from build123d import *

# Parameters (mm, degrees)
F1_DEPTH  = 25.4
F2_R      = 3.556
F3_DEPTH  = 30.342798
F3_FACE_R = 3.556
F4_DEPTH  = 45.857202


with BuildPart() as f1:
    # F0 (on Top) → F1 (new body)
    with BuildSketch(Plane.XY):
        with BuildLine():
            Line((-2.147933, 7.757202), (-29.198933, 7.757202))
            Line((-29.198933, 7.757202), (-29.198933, -30.342798))
            Line((-29.198933, -30.342798), (66.051067, -30.342798))
            Line((66.051067, -30.342798), (66.051067, 7.757202))
            Line((66.051067, 7.757202), (45.350067, 7.757202))
            ThreePointArc((45.350067, 7.757202), (21.601067, -15.991798), (-2.147933, 7.757202))
        make_face()
        with BuildLine():
            Line((66.051067, 45.857202), (-29.198933, 45.857202))
            Line((-29.198933, 45.857202), (-29.198933, 7.757202))
            Line((-29.198933, 7.757202), (-2.147933, 7.757202))
            ThreePointArc((-2.147933, 7.757202), (21.601067, 31.506202), (45.350067, 7.757202))
            Line((45.350067, 7.757202), (66.051067, 7.757202))
            Line((66.051067, 7.757202), (66.051067, 45.857202))
        make_face()
    extrude(amount=F1_DEPTH)

    # F2 (on Front) → F3 (cut, through all)
    with BuildSketch(Plane.XZ):
        with Locations((-19.768986, 12.707096)):
            Circle(F2_R)
        with Locations((56.431014, 12.707096)):
            Circle(F2_R)
    extrude(amount=F3_DEPTH, mode=Mode.SUBTRACT)

    # F3_face (on face) → F4 (cut, through all)
    with BuildSketch(Plane(origin=(-19.768986, 0, 12.707096), x_dir=(1, 0, 0), z_dir=(0, -1, 0))):
        Circle(F3_FACE_R)
        with Locations((76.2, 0)):
            Circle(F3_FACE_R)
    extrude(amount=-F4_DEPTH, mode=Mode.SUBTRACT)


solid = f1.part
Work out the finished part from the listing and answer in its coordinate system (mm). Give positions to 0.01 mm unless a question says otherwise; leave off trailing zeros. Order: outer loops, then holes, each group sorted by start corner. A loop starts at its lowest first (then second) coordinate and runs counter-clockwise, first axis right, second up. Notation, with made-up numbers: (56.5, -38.75) - (115.5, -38.75) arc R21 ccw to (115.5, -30.75) - close; hole circle Ø5 at (53.25, 70.5). An arc over 180 degrees is marked (long way). Answer as CSV lines item,"result". Start each with the question number.
Q1. Find the intervals of material crossed by L1, parallel to X at y = -4, z = 12.25; L2, parallel to X at y = -8, z = 17.25; L3, parallel to X at y = -13.5, z = 2.5, in increasing order. Write a range as [from, to].
Q2. The part is cut by section C-C (x = 32.5). Write down the section's boundary in (y, z).
Q3. The mould has two halves that part along X. Classify faces 1 (the face through (66.051, 7, 13)), 2 (the face through (19, 45.857, 13)), 3 (the face through (59.82, 8.29, 13.78)): +X half, -X half, draft (parallel to the pull), parting line (faces both ways), or undercut.
Q4. The part is cut by section D-D (y = 15). Write down the section's boundary in (x, z), then the cut area to 3 significant figures.
Q5. Given pin 1 Ø4.5 at (x, z) = (-19.77, 12.71) entering from +Y, flat-ended and moving along its own axis, determine where the tip first touches the part or whether it passes through.
Q6. The part is cut by section A-A (y = 6.5). Write down the section's boundary in (x, z).
Q7. The part is cut by section B-B (z = 14). Write down the section's boundary in (x, y).
Check result:
1,L1,"x = [-29.2, -23.3], [-16.24, 0.97], [42.24, 52.9], [59.96, 66.05]"
1,L2,"x = [-29.2, 3.83], [39.37, 66.05]"
1,L3,"x = [-29.2, 11.01], [32.19, 66.05]"
2,outline,"(-30.34, 0) - (-13.34, 0) - (-13.34, 25.4) - (-30.34, 25.4) - close; (28.86, 0) - (45.86, 0) - (45.86, 25.4) - (28.86, 25.4) - close"
3,face 1,"+X half"
3,face 2,"draft"
3,face 3,"undercut"
4,outline,"(-29.2, 0) - (-1.02, 0) - (-1.02, 25.4) - (-29.2, 25.4) - close; (44.22, 0) - (66.05, 0) - (66.05, 25.4) - (44.22, 25.4) - close; hole circle Ø7.11 at (-19.77, 12.71); hole circle Ø7.11 at (56.43, 12.71)"
4,area,"1,190 mm²"
5,pin 1,"passes through"
6,outline,"(-29.2, 0) - (-2.11, 0) - (-2.11, 25.4) - (-29.2, 25.4) - close; (45.32, 0) - (66.05, 0) - (66.05, 25.4) - (45.32, 25.4) - close; hole circle Ø7.11 at (-19.77, 12.71); hole circle Ø7.11 at (56.43, 12.71)"
7,outline,"(-29.2, -30.34) - (-23.08, -30.34) - (-23.08, 45.86) - (-29.2, 45.86) - close; (-16.46, -30.34) - (53.12, -30.34) - (53.12, 45.86) - (-16.46, 45.86) - close; (59.74, -30.34) - (66.05, -30.34) - (66.05, 45.86) - (59.74, 45.86) - close; hole circle Ø47.5 at (21.6, 7.76)"
